CAD build for the part. Positions are in the model's coordinates, mm. A direction names the side the tool comes from. Give positions to 0.01 mm unless a question says otherwise; leave off trailing zeros. Order: outer loops, then holes, each group sorted by start corner. A loop starts at its lowest first (then second) coordinate and runs counter-clockwise, first axis right, second up.
Item 1: Band-saw the part on C-C on y = -1.5. Give the cut face in (x, z).
Item 2: Wall check: L1, parallel to Y at x = 0.25, z = 0.5; L2, parallel to Y at x = 6.75, z = -3.6; L3, parallel to Z at x = 8, y = 0. Give the ranges that are in metal, low to high.
Item 3: Band-saw the part on A-A on x = 0.5. Give the cut face in (y, z).
Item 4: Which spindle directions (+Z, -Z, +X, -X, +Y, -Y) get a long thin tool onto all of the face, cutting with end or side? Do faces 1 (the flat face through (0, 3, -5)), 2 (the flat face through (-6.48, 1.27, 0.07)), 3 (the cylindrical face through (7.285, -1.13, -2.725)). Say none if no direction does.
Item 5: Flat gauge pins, fed straight in: P1, Ø1.8, axis at x = 6.75, y = 0, coming from the -Z side; P2, Ø4.5, axis at y = -1, z = 1, coming from the +X side. Where does each tip first touch, or does it go through?
Item 6: Two-plate mould, pull along X, no slides. Class faces 4 (the flat face through (0, -5.5, 0)), 5 (the flat face through (4.75, 0, 0)), 6 (the cylindrical face through (6.88, 0.99, 3.87)): released by +X, released by -X, zero draft, split by the parting line, or undercut.
Item 7: Band-saw the part on B-B on z = 0. Give the cut face in (x, y), plus the area to 3 significant figures.
Item 8: Band-saw the part on D-D on x = 8.25. Give the cut face in (y, z), plus the area to 3 significant figures.
```python
from build123d import *

# Parameters (mm, degrees)
SKETCH_1_W            = 19.5
SKETCH_1_H            = 11
EXTRUDE_1_DEPTH       = 5
SKETCH_2_R            = 2.95
CUT_EXTRUDE_1_DEPTH   = 5
HOLE_WIZARD_2_0_2_1_D = 2


with BuildPart() as part:
    # 草图1 → 凸台-拉伸1 (new, symmetric)
    with BuildSketch(Plane.XY):
        Rectangle(SKETCH_1_W, SKETCH_1_H)
        with BuildLine():
            Line((-5.25, 2.5), (-7.75, 0))
            Line((-7.75, 0), (-5.25, -2.5))
            Line((-5.25, -2.5), (1.25, -2.5))
            ThreePointArc((1.25, -2.5), (3.75, 0), (1.25, 2.5))
            Line((1.25, 2.5), (-5.25, 2.5))
        make_face(mode=Mode.SUBTRACT)
    extrude(amount=EXTRUDE_1_DEPTH, both=True)

    # 草图2 → 切除-拉伸1 (cut)
    with BuildSketch(Plane(origin=(9.75, 0, 0), x_dir=(0, 0, -1), z_dir=(1, 0, 0))):
        Circle(SKETCH_2_R)
    extrude(amount=-CUT_EXTRUDE_1_DEPTH, mode=Mode.SUBTRACT)

    # Ø2.0 (2) 直径孔1 (through all)
    with Locations(Plane.XY.offset(5)):
        with Locations((6.75, 0)):
            Hole(HOLE_WIZARD_2_0_2_1_D / 2)


solid = part.part
```
The answers:
1. outline: (-9.75, -5) - (-6.25, -5) - (-6.25, 5) - (-9.75, 5) - close; (3.25, -5) - (9.75, -5) - (9.75, -2.54) - (4.75, -2.54) - (4.75, 2.54) - (9.75, 2.54) - (9.75, 5) - (3.25, 5) - close
2. L1: y = -5.5 to -2.5, 2.5 to 5.5
2. L2: y = -5.5 to -1, 1 to 5.5
2. L3: z = -5 to -2.95, 2.95 to 5
3. outline: (-5.5, -5) - (-2.5, -5) - (-2.5, 5) - (-5.5, 5) - close; (2.5, -5) - (5.5, -5) - (5.5, 5) - (2.5, 5) - close
4. face 1: -Z, +X, -X, +Y, -Y
4. face 2: +Z, -Z
4. face 3: +X
5. P1: passes through
5. P2: stops at x = 9.75
6. face 4: zero draft
6. face 5: released by +X
6. face 6: undercut
7. outline: (-9.75, -5.5) - (9.75, -5.5) - (9.75, -2.95) - (4.75, -2.95) - (4.75, 2.95) - (9.75, 2.95) - (9.75, 5.5) - (-9.75, 5.5) - close; hole (-7.75, 0) - (-5.25, -2.5) - (1.25, -2.5) arc R2.5 ccw to (1.25, 2.5) - (-5.25, 2.5) - close
7. area: 136 mm2
8. outline: (-5.5, -5) - (5.5, -5) - (5.5, 5) - (-5.5, 5) - close; hole circle Ø5.9 at (0, 0)
8. area: 82.7 mm2
